from build123d import *

# Parameters (mm, degrees)
F0_R     = 50.8
F1_DEPTH = 12.7
F4_DEPTH = 25.4
F5_R     = 37.465
F5_R_2   = 31.75
F6_DEPTH = 76.2
F8_ANGLE = 15.83


with BuildPart() as f1:
    # F0 (on Front) → F1 (new body)
    with BuildSketch(Plane.XZ):
        Circle(F0_R)
    extrude(amount=F1_DEPTH)

    # F2 (on Right) → F3 (revolve, cut)
    with BuildSketch(Plane.YZ):
        Polygon((-12.895335, -50.86495), (0, -51.151514), (-12.895335, -36.823358), align=None)
    revolve(axis=Axis((0, 0, 0), (0, 1, 0)), mode=Mode.SUBTRACT)

    # F2 (on Right) → F4 (cut)
    with BuildSketch(Plane.YZ):
        Polygon((-12.895335, -50.86495), (0, -51.151514), (-12.895335, -36.823358), align=None)
    extrude(amount=-F4_DEPTH, mode=Mode.SUBTRACT)

    # F5 (on Front) → F6 (join)
    with BuildSketch(Plane.XZ):
        Circle(F5_R)
        Circle(F5_R_2, mode=Mode.SUBTRACT)
    extrude(amount=-F6_DEPTH)

    # F7 (on Top) → F8 (revolve)
    with BuildSketch(Plane.XY):
        Polygon((-37.465, -0.075845), (-37.465, 18.974155), (-44.45, 14.211659), (-44.45, 4.686659), align=None)
        Polygon((-37.465, 18.974155), (-37.465, 38.024155), (-44.45, 33.261659), (-44.45, 23.736659), align=None)
        Polygon((-37.465, 38.024155), (-37.465, 57.074155), (-44.45, 52.311659), (-44.45, 42.786659), align=None)
        Polygon((-37.465, 57.074155), (-37.465, 76.124155), (-44.45, 71.361659), (-44.45, 61.836659), align=None)
    revolve(axis=Axis((0, 76.2, 0), (0, -1, 0)), revolution_arc=F8_ANGLE)


solid = f1.part
Part model, mm, in its own coordinate system. A direction names the side the tool comes from. Give positions to 0.01 mm unless a question says otherwise; leave off trailing zeros. Loops run counter-clockwise (first coordinate to the right, second up) from the corner with the lowest first, then second, coordinate; pieces in that order, holes last.
(1) Band-saw the part on C-C (y = 55). Write the cut outline in (x, z) (3 decimals), and give its area (3 significant figures).
Return value:
outline: (-40.507, 0) arc R40.507 ccw to (-38.971, -11.05) - (-36.044, -10.22) arc R37.465 ccw (long way) to (-37.465, 0) - close; hole circle Ø63.5 at (0, 0)
area: 1,280 mm2
(2) Band-saw the part on B-B (y = 8). Write the cut outline in (x, z) (3 decimals).
Return value:
outline: (-44.45, 0) arc R44.45 ccw to (-42.764, -12.125) - (-36.044, -10.22) arc R37.465 ccw (long way) to (-37.465, 0) - close; hole circle Ø63.5 at (0, 0)
(3) Drill centre lines: line 1 along Z through (x, y) = (0, 41.5) (3 decimals); line 2 along X through (y, z) = (10, -29); line 3 along Z through (x, y) = (13, 9). Where is each one in solid material? Low to high.
Return value:
line 1: z = -37.465 to -31.75, 31.75 to 37.465
line 2: x = -23.72 to -12.93, 12.93 to 23.72
line 3: z = -35.14 to -28.97, 28.97 to 35.14
(4) 3-axis set-ups, long thin cutter, end or side, ignore diameter. For faces 1 (the cylindrical face through (-44.038, 47.482, -6.036)), 2 (the flat face through (-38.705, 47.683, -10.974)), 3 (the flat face through (-40, 67, 0)), 4 (the cylindrical face through (-29.73, 37.57, -22.8)): which of +Z, -Z, +X, -X, +Y, -Y reach the whole face in a straight line?
Return value:
face 1: -Z, -X, +Y
face 2: -Z, +Y
face 3: +Z, -X, +Y
face 4: +Y
(5) Pin check, flat tips, straight feed: pin 1 (2 mm diameter, centred on x = -39.5, y = 66.5, fed in from +Z); pin 2 (1.5 mm diameter, centred on x = -19, y = 54.5, fed in from +Z); pin 3 (6 mm diameter, centred on x = -26.5, y = 21.5, fed in from +Z). Stop position of each tip, or through.
Return value:
pin 1: stops at z = 0
pin 2: stops at z = 32.72
pin 3: stops at z = 29.18
(6) Pull direction X, two halves, no side cores. Call faces 5 (the conical face through (-40.627, 73.71, -5.568)), 6 (the cylindrical face through (-11.012, -0.156, -49.592)), 7 (the flat face through (-38.705, 9.62, -10.974)), 8 (the flat face through (-40, 29, 0)): pulls with the +X half, pulls with the -X half, needs draft (parallel to the pull), parting line crosses it, or undercut.
Return value:
face 5: pulls with the -X half
face 6: parting line crosses it
face 7: undercut
face 8: needs draft
(7) Band-saw the part on A-A (x = 0). Write the cut outline in (y, z) (3 decimals).
Return value:
outline: (-12.7, -37.04) - (-0.316, -50.8) - (0, -50.8) - (0, -37.465) - (76.2, -37.465) - (76.2, -31.75) - (0, -31.75) - (0, 31.75) - (76.2, 31.75) - (76.2, 37.465) - (0, 37.465) - (0, 50.8) - (-0.316, 50.8) - (-12.7, 37.04) - close
